Drawing for the job (mm, zero at the part's lowest x, y, z). Give positions to 0.01 mm unless a question says otherwise; leave off trailing zeros. Order: outer loops, then holes, each group sorted by start corner. A loop starts at its lowest first (then second) coordinate and runs counter-clockwise, first axis right, second up. Notation, with made-up numbers: (75, 1) - (81, 1) arc R13 ccw to (81, 23) - close; hole circle Ø6 at (39, 51). An arc over 180 degrees is marked (long way). Use a Markdown table: item, result. Add a question column.
(1) Slice it at C-C (z = 2.5). Write the cut outline in (x, y), then the cut area to 3 significant figures.
(2) Mould opens along Y. For the marked faces 1, 2 and 3 say: +Y half, -Y half, draft (parallel to the pull), parting line (faces both ways), or undercut.
(3) Flat gauge pins, fed straight in: pin 1 (12 mm diameter, centred on x = 25.5, y = 6, fed in from -Z); pin 2 (5 mm diameter, centred on x = 25.5, z = 10.5, fed in from -Y); pin 3 (1 mm diameter, centred on y = 7.5, z = 4.5, fed in from -X); pin 4 (2 mm diameter, centred on y = 15, z = 18, fed in from -X). Where does each tip first touch, or does it go through?
(4) Slice it at A-A (y = 15). Write the cut outline in (x, z).
(5) Wall check: line 1 (Y direction, x = 15, z = 9.75); line 2 (Y direction, x = 9.25, z = 16.75); line 3 (Z direction, x = 17, y = 2.25). Give the ranges that are in metal, low to high.
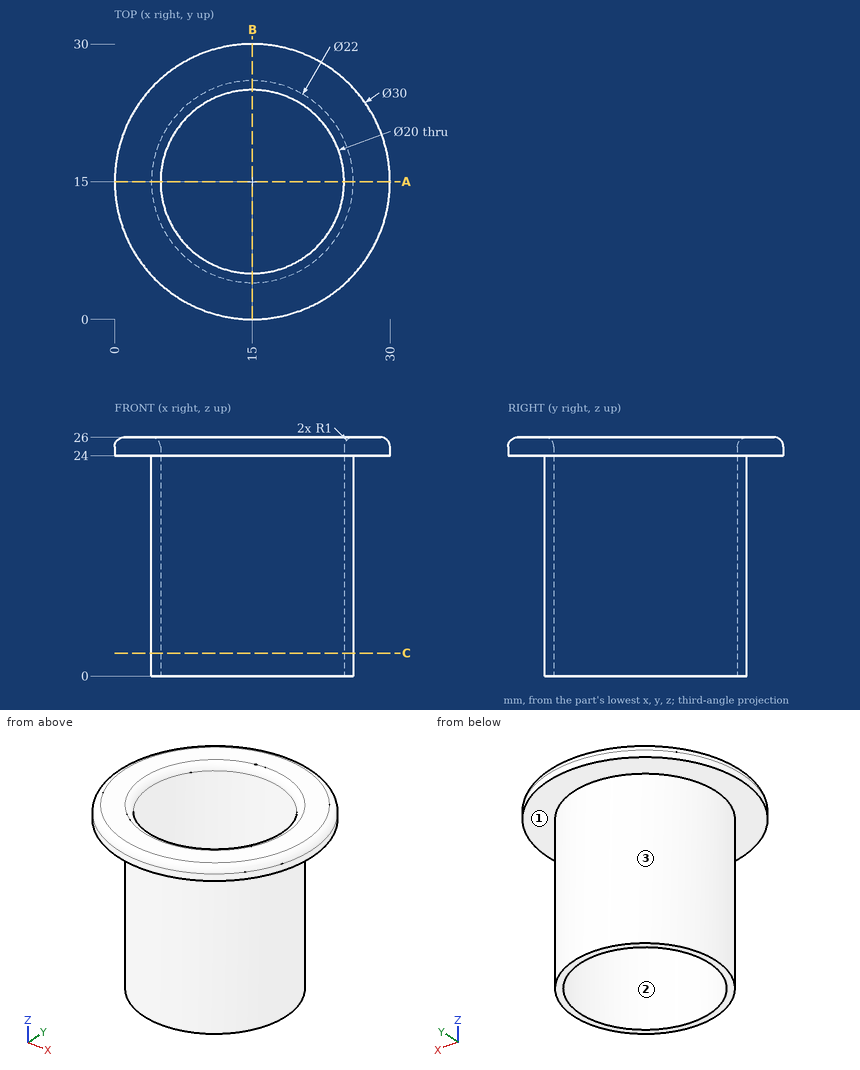
Solution:
| question | item | result |
|---|---|---|
| 1 | outline | circle Ø22 at (15, 15); hole circle Ø20 at (15, 15) |
| 1 | area | 66.0 mm2 |
| 2 | face 1 | draft |
| 2 | face 2 | undercut |
| 2 | face 3 | parting line |
| 3 | pin 1 | z = 0 |
| 3 | pin 2 | y = 7.45 |
| 3 | pin 3 | x = 6.51 |
| 3 | pin 4 | x = 4 |
| 4 | outline | (0, 24) - (4, 24) - (4, 0) - (5, 0) - (5, 25) arc R1 ccw to (4, 26) - (1, 26) arc R1 ccw to (0, 25) - close; (25, 0) - (26, 0) - (26, 24) - (30, 24) - (30, 25) arc R1 ccw to (29, 26) - (26, 26) arc R1 ccw to (25, 25) - close |
| 5 | line 1 | 4 to 5, 25 to 26 |
| 5 | line 2 | 5.62 to 6.82, 23.18 to 24.38 |
| 5 | line 3 | 24 to 26 |
